from build123d import *

# Parameters (mm, degrees)
F1_DEPTH = 50
F2_R     = 18
F3_DEPTH = 60
F4_W     = 40
F4_H     = 26
F5_DEPTH = 25
F7_DEPTH = 30
F8_R     = 11
F9_DEPTH = 40


# Not quite as in the source:
# - a feature names something its author has since deleted; it is built from what else it names


with BuildPart() as f1:
    # F0 (on Front) → F1 (new body)
    with BuildSketch(Plane.XZ):
        Polygon((-60, 12.5), (-60, -12.5), (60, -12.5), (60, 12.5), (30, 12.5), (-30, 12.5), align=None)
    extrude(amount=F1_DEPTH)

    # F2 (on face) → F3 (cut)
    with BuildSketch(Plane.XZ.offset(50)):
        with Locations((0, -12.5)):
            Circle(F2_R)
    extrude(amount=-F3_DEPTH, mode=Mode.SUBTRACT)

    # F4 (on face) → F5 (cut)
    with BuildSketch(Plane.XY.offset(12.5)):
        with Locations((-60, -25)):
            Rectangle(F4_W, F4_H)
        with Locations((60, -25)):
            Rectangle(F4_W, F4_H)
    extrude(amount=-F5_DEPTH, mode=Mode.SUBTRACT)

    # F6 (on face) → F7 (join)
    with BuildSketch(Plane.XY.offset(12.5)):
        Polygon((30, -25), (0, 0), (-30, -25), (0, -50), align=None)
    extrude(amount=F7_DEPTH)

    # F8 (on face) → F9 (cut)
    with BuildSketch(Plane.XY.offset(42.5)):
        with Locations((0, -25)):
            Circle(F8_R)
    extrude(amount=-F9_DEPTH, mode=Mode.SUBTRACT)


solid = f1.part
Build history of the part. All positions in model axes, mm. A direction names the side the tool comes from. Round coordinates to 2 decimals unless told otherwise and drop trailing zeros. Write each loop counter-clockwise with the first axis right and the second up, starting at its lowest first coordinate (ties: lowest second). Pieces come first, ordered by that corner, then holes. Notation, with made-up numbers: (-23, -21) -> (17, -21) arc R10 ccw to (17, -4) -> close; hole circle Ø11 at (74.5, 74). An arc over 180 degrees is marked (long way). Write item = value, one per line.
(1) Band-saw the part on D-D (y = -44). Give the cut face in (x, z), then the cut area to 3 significant figures.
Answer:
outline = (-60, -12.5) -> (-18, -12.5) arc R18 cw to (18, -12.5) -> (60, -12.5) -> (60, 12.5) -> (7.2, 12.5) -> (7.2, 42.5) -> (-7.2, 42.5) -> (-7.2, 12.5) -> (-60, 12.5) -> close
area = 2,920 mm2
(2) Tool access for faces 1 (the face through (14.79, -37.675, 27.29)), 2 (the face through (15.21, -12.675, 27.29)), 3 (the face through (50, -38, 0)): list every direction of +Z, -Z, +X, -X, +Y, -Y with a clear straight run to the whole face (end or side of a thin tool).
Answer:
face_1 = +Z, +X, -Y
face_2 = +Z, +X, +Y
face_3 = +Z, -Z, +X
(3) Band-saw the part on A-A (x = 43.5). Give the cut face in (y, z), then the cut area to 3 significant figures.
Answer:
outline = (-50, -12.5) -> (-38, -12.5) -> (-38, 12.5) -> (-50, 12.5) -> close; (-12, -12.5) -> (0, -12.5) -> (0, 12.5) -> (-12, 12.5) -> close
area = 600 mm2
(4) Band-saw the part on B-B (z = 8.5). Give the cut face in (x, y), then the cut area to 3 significant figures.
Answer:
outline = (-60, -50) -> (60, -50) -> (60, -38) -> (40, -38) -> (40, -12) -> (60, -12) -> (60, 0) -> (-60, 0) -> (-60, -12) -> (-40, -12) -> (-40, -38) -> (-60, -38) -> close; hole circle Ø22 at (0, -25)
area = 4,580 mm2
(5) Band-saw the part on C-C (y = -23). Give the cut face in (x, z), then the cut area to 3 significant figures.
Answer:
outline = (-40, -12.5) -> (-18, -12.5) arc R18 cw to (-9.95, 2.5) -> (-10.82, 2.5) -> (-10.82, 42.5) -> (-27.6, 42.5) -> (-27.6, 12.5) -> (-40, 12.5) -> close; (9.95, 2.5) arc R18 cw to (18, -12.5) -> (40, -12.5) -> (40, 12.5) -> (27.6, 12.5) -> (27.6, 42.5) -> (10.82, 42.5) -> (10.82, 2.5) -> close
area = 2,320 mm2
(6) Two-plate mould, pull along Y, no slides. Class faces 4 (the face through (-14.79, -12.325, 27.29)), 5 (the face through (-40, -25, 0)), 6 (the face through (50, -12, 0)), 7 (the face through (-15.21, -37.325, 27.29)): pulls with the +Y half, pulls with the -Y half, needs draft (parallel to the pull), parting line crosses it, or undercut.
Answer:
face_4 = pulls with the +Y half
face_5 = undercut
face_6 = undercut
face_7 = pulls with the -Y half
(7) Flat gauge pins, fed straight in: pin 1 (15 mm diameter, centred on x = 39.5, y = -37.5, fed in from +Z); pin 2 (3 mm diameter, centred on y = -17.5, z = 7.5, fed in from +X); pin 3 (8 mm diameter, centred on x = 18.5, z = 33, fed in from -Y). Where does each tip first touch, or does it go through?
Answer:
pin_1 = 12.5
pin_2 = 40
pin_3 = -37.92
(8) Probe L1, parallel to Y at x = -44.5, z = 7; L2, parallel to Y at x = 0, z = 34; L3, parallel to X at y = -25, z = 16.5. List the from-to ranges inside material, lowest first.
Answer:
L1 = -50 to -38, -12 to 0
L2 = -50 to -36, -14 to 0
L3 = -30 to -11, 11 to 30
